Input: dimensioned drawing with shaded views. Units: mm. Origin: part minimum x, y, z. Give positions to 0.01 mm unless a question says otherwise; leave off trailing zeros. Loops run counter-clockwise (first coordinate to the right, second up) from the corner with the lowest first, then second, coordinate; pieces in that order, holes last. Notation, with made-up numbers: (-25.75, -26.5) -> (24.25, -26.5) arc R16 ccw to (24.25, 4.5) -> close; hole circle Ø7 at (60.25, 49). An arc over 180 degrees is marked (long way). Answer as a JSON object with one key per item and string values.
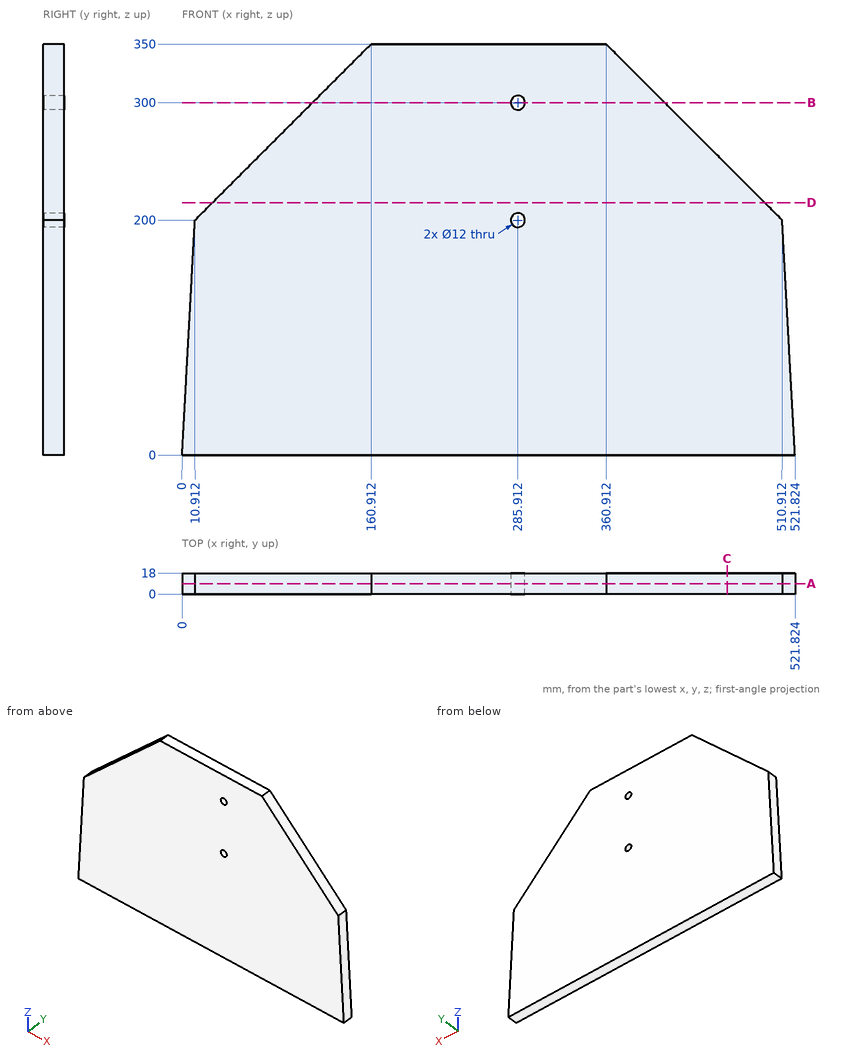
Q1. Ray query, line 1 along Z through (x, y) = (287.5, 12.5) (1 decimal); line 2 along X through (y, z) = (6.75, 300); line 3 along Z through (x, y) = (473, 5.5). Return the intervals inside material, ascending.
Evaluation:
{"line 1": "z = 0 to 194.2, 205.8 to 294.2, 305.8 to 350", "line 2": "x = 110.91 to 279.91, 291.91 to 410.91", "line 3": "z = 0 to 237.91"}
Q2. Section B-B, the plane z = 300. Return the cut outline in (x, y), then the cut area to 3 significant figures.
Evaluation:
{"outline": "(110.91, 0) -> (279.91, 0) -> (279.91, 18) -> (110.91, 18) -> close; (291.91, 0) -> (410.91, 0) -> (410.91, 18) -> (291.91, 18) -> close", "area": "5,180 mm2"}
Q3. Section D-D, the plane z = 215. Return the cut outline in (x, y), then the cut area to 3 significant figures.
Evaluation:
{"outline": "(25.91, 0) -> (495.91, 0) -> (495.91, 18) -> (25.91, 18) -> close", "area": "8,460 mm2"}
Q4. Section C-C, the plane x = 464. Return the cut outline in (y, z), then the cut area to 3 significant figures.
Evaluation:
{"outline": "(0, 0) -> (18, 0) -> (18, 246.91) -> (0, 246.91) -> close", "area": "4,440 mm2"}
Q5. Pin query (flat end, axial travel): pin 1 (8 mm diameter, centred on y = 4.5, z = 38.5, fed in from +X); pin 2 (10 mm diameter, centred on x = 390, y = 5.5, fed in from +Z); pin 3 (4 mm diameter, centred on x = 106.5, y = 6.5, fed in from +Z). Return the tip coordinate at first contact, or that it passes through.
Evaluation:
{"pin 1": "stops at x = 519.94", "pin 2": "stops at z = 325.91", "pin 3": "stops at z = 297.59"}
Q6. Section A-A, the plane y = 9. Return the cut outline in (x, z), then the cut area to 3 significant figures.
Evaluation:
{"outline": "(0, 0) -> (521.82, 0) -> (510.91, 200) -> (360.91, 350) -> (160.91, 350) -> (10.91, 200) -> close; hole circle Ø12 at (285.91, 200); hole circle Ø12 at (285.91, 300)", "area": "154,000 mm2"}
